```python
from build123d import *

# Parameters (mm, degrees)
EXTRUDE_1_DEPTH     = 10
CUT_EXTRUDE_3_DEPTH = 16
SKETCH_6_W          = 4
SKETCH_6_H          = 3.2
SKETCH_6_W_2        = 3.2
SKETCH_6_H_2        = 4
CUT_EXTRUDE_5_DEPTH = 6.5
SKETCH_7_W          = 6
SKETCH_7_H          = 3
SKETCH_7_W_2        = 3
SKETCH_7_H_2        = 6
CUT_EXTRUDE_6_DEPTH = 16.5
SKETCH_8_W          = 40
SKETCH_8_H          = 20
EXTRUDE_2_DEPTH     = 10
SKETCH_9_W          = 41
SKETCH_9_H          = 10
EXTRUDE_3_DEPTH     = 23.36
SKETCH_10_W         = 41
SKETCH_10_H         = 8
EXTRUDE_4_DEPTH     = 40
SKETCH_11_W         = 8
SKETCH_11_H         = 8
EXTRUDE_5_DEPTH     = 10
SKETCH_12_R         = 2.5
CUT_EXTRUDE_7_DEPTH = 10
FILLET_1_R          = 20
FILLET_2_R          = 15


with BuildPart() as part:
    # 草图1 → 凸台-拉伸1 (new body)
    with BuildSketch(Plane(origin=(0, 0, 0), x_dir=(1, 0, 0), z_dir=(0, 1, 0))):
        Polygon((0, 105), (0, 75), (0, 0), (30, 0), (30, 75), (41, 75), (41, 105), (30, 105), align=None)
    extrude(amount=EXTRUDE_1_DEPTH)

    # 草图4 → 切除-拉伸3 (cut)
    with BuildSketch(Plane(origin=(0, 10, 0), x_dir=(1, 0, 0), z_dir=(0, 1, 0))):
        with BuildLine():
            Line((12, 15), (12, 76.76156826))
            ThreePointArc((12, 76.76156826), (15, 79.76156826), (18, 76.76156826))
            Line((18, 76.76156826), (18, 15))
            ThreePointArc((18, 15), (15, 12), (12, 15))
        make_face()
    extrude(amount=-CUT_EXTRUDE_3_DEPTH, mode=Mode.SUBTRACT)

    # 草图6 → 切除-拉伸5 (cut)
    with BuildSketch(Plane(origin=(0, 10, 0), x_dir=(1, 0, 0), z_dir=(0, 1, 0))):
        with Locations((39, 100)):
            Rectangle(SKETCH_6_W, SKETCH_6_H)
        with Locations((5, 2)):
            Rectangle(SKETCH_6_W_2, SKETCH_6_H_2)
        with Locations((39, 90)):
            Rectangle(SKETCH_6_W, SKETCH_6_H)
        with Locations((39, 80)):
            Rectangle(SKETCH_6_W, SKETCH_6_H)
        with Locations((15, 2)):
            Rectangle(SKETCH_6_W_2, SKETCH_6_H_2)
        with Locations((25, 2)):
            Rectangle(SKETCH_6_W_2, SKETCH_6_H_2)
    extrude(amount=-CUT_EXTRUDE_5_DEPTH, mode=Mode.SUBTRACT)

    # 草图7 → 切除-拉伸6 (cut)
    with BuildSketch(Plane(origin=(0, 10, 0), x_dir=(1, 0, 0), z_dir=(0, 1, 0))):
        with Locations((5, 5.5)):
            Rectangle(SKETCH_7_W, SKETCH_7_H)
        with Locations((15, 5.5)):
            Rectangle(SKETCH_7_W, SKETCH_7_H)
        with Locations((25, 5.5)):
            Rectangle(SKETCH_7_W, SKETCH_7_H)
        with Locations((35.5, 100)):
            Rectangle(SKETCH_7_W_2, SKETCH_7_H_2)
        with Locations((35.5, 90)):
            Rectangle(SKETCH_7_W_2, SKETCH_7_H_2)
        with Locations((35.5, 80)):
            Rectangle(SKETCH_7_W_2, SKETCH_7_H_2)
    extrude(amount=-CUT_EXTRUDE_6_DEPTH, mode=Mode.SUBTRACT)

    # 草图8 → 凸台-拉伸2 (add)
    with BuildSketch(Plane.XZ):
        with Locations((50, -65)):
            Rectangle(SKETCH_8_W, SKETCH_8_H)
    extrude(amount=-EXTRUDE_2_DEPTH)

    # 草图9 → 凸台-拉伸3 (add)
    with BuildSketch(Plane(origin=(0, 0, -105), x_dir=(-1, 0, 0), z_dir=(0, 0, -1))):
        with Locations((-20.5, 5)):
            Rectangle(SKETCH_9_W, SKETCH_9_H)
    extrude(amount=EXTRUDE_3_DEPTH)

    # 草图10 → 凸台-拉伸4 (add)
    with BuildSketch(Plane(origin=(0, 10, 0), x_dir=(1, 0, 0), z_dir=(0, 1, 0))):
        with Locations((20.5, 124.36)):
            Rectangle(SKETCH_10_W, SKETCH_10_H)
    extrude(amount=EXTRUDE_4_DEPTH)

    # 草图11 → 凸台-拉伸5 (add)
    with BuildSketch(Plane.XZ):
        with Locations((34, -4)):
            Rectangle(SKETCH_11_W, SKETCH_11_H)
    extrude(amount=-EXTRUDE_5_DEPTH)

    # 草图12 → 切除-拉伸7 (cut)
    with BuildSketch(Plane(origin=(0, 0, -8), x_dir=(-1, 0, 0), z_dir=(0, 0, -1))):
        with Locations((-34, 5)):
            Circle(SKETCH_12_R)
    extrude(amount=-CUT_EXTRUDE_7_DEPTH, mode=Mode.SUBTRACT)

    # 圆角1
    fillet_1_edges = [part.edges().sort_by_distance(p)[0] for p in [
        (30, 5, -55),
    ]]
    fillet(fillet_1_edges, radius=FILLET_1_R)

    # 圆角2
    fillet_2_edges = [part.edges().sort_by_distance(p)[0] for p in [
        (20.5, 10, -120.36),
    ]]
    fillet(fillet_2_edges, radius=FILLET_2_R)


solid = part.part
```
Check sheet for the modelled part. Datum: model origin and axes. Units: mm. A direction names the side the tool comes from. Coordinates: 2 decimals unless noted, no trailing zeros. Write each loop counter-clockwise with the first axis right and the second up, starting at its lowest first coordinate (ties: lowest second). Pieces come first, ordered by that corner, then holes. Notation, with made-up numbers: (-37, -23) - (-5, -23) arc R17 ccw to (-5, -7) - close; hole circle Ø11 at (-3, 63). An arc over 180 degrees is marked (long way). One line per question, with ' | ' between items.
Item 1: Mould release check, pull along Z, two halves, no side actions. Record for faces 5 (the face through (25, 5, -7)), 6 (the face through (60, 5, -55)), 7 (the face through (41, 12, -115)): pulls with the +Z half, pulls with the -Z half, needs draft (parallel to the pull), parting line crosses it, or undercut.
Determined:
face 5: undercut | face 6: pulls with the +Z half | face 7: needs draft
Item 2: Thickness scan on line 1 (Y direction, x = 34, z = -1); line 2 (Z direction, x = 10, y = 32); line 3 (Y direction, x = 46.5, z = -56). Record the ranges inside material, lowest first. Write a range as [from, to].
Determined:
line 1: y = [0, 2.5], [7.5, 10] | line 2: z = [-128.36, -120.36] | line 3: y = [0, 10]
Item 3: Sectioned sample at B-B on x = 15. Record the boundary of the cut face in (y, z), plus the area to 3 significant figures.
Determined:
outline: (0, -128.36) - (50, -128.36) - (50, -120.36) - (25, -120.36) arc R15 cw to (10, -105.36) - (10, -79.76) - (0, -79.76) - close; (0, -12) - (10, -12) - (10, -7) - (0, -7) - close; (0, -4) - (3.5, -4) - (3.5, 0) - (0, 0) - close | area: 918 mm2
Item 4: Sectioned sample at D-D on y = 43.5. Record the boundary of the cut face in (x, z).
Determined:
outline: (0, -128.36) - (41, -128.36) - (41, -120.36) - (0, -120.36) - close
Item 5: Sectioned sample at A-A on z = -21. Record the boundary of the cut face in (x, y), plus the area to 3 significant figures.
Determined:
outline: (0, 0) - (12, 0) - (12, 10) - (0, 10) - close; (18, 0) - (30, 0) - (30, 10) - (18, 10) - close | area: 240 mm2
Item 6: Sectioned sample at C-C on y = 5. Give the number of separate pieces and of enclosed holes in the cut face, plus the area to 3 significant figures.
Determined:
separate pieces: 2 | enclosed holes: 1 | area: 4,760 mm2
Item 7: Gauge pin test, flat ends, axial feed: P1, Ø3, axis at x = 20, y = 44.5, coming from the +Z side; P2, Ø1.2, axis at y = 5, z = -2.5, coming from the -X side; P3, Ø5, axis at x = 38.5, z = -113, coming from the +Y side; P4, Ø1, axis at x = 16.5, y = 13.5, coming from the +Z side. Record the tip position at first contact, or that the pin passes through.
Determined:
P1: stops at z = -120.36 | P2: stops at x = 0 | P3: stops at y = 13.95 | P4: stops at z = -114.36
Item 8: Access from +Z, -Z, +X, -X, +Y, -Y to the whole of each face (thin tool, end or side, straight path). Record for faces 1 (the face through (70, 5, -65)), 2 (the face through (39, 7, -88.4)), 3 (the face through (19, 10, -52)), 4 (the face through (15, 5, -12)).
Determined:
face 1: +Z, -Z, +X, +Y, -Y | face 2: +X, +Y | face 3: +Z, +X, -X, +Y | face 4: +Y, -Y
